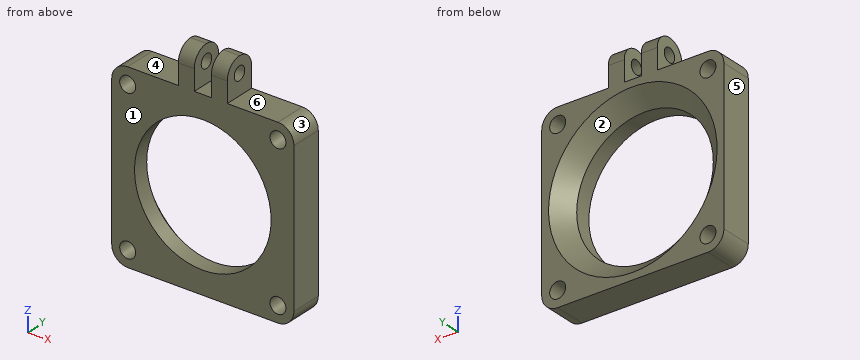
from build123d import *

# Parameters (mm, degrees)
BOSS_EXTRUDE1_DEPTH = 7
CUT_EXTRUDE2_REACH  = 31.138
SKETCH3_R           = 1.75
SKETCH7_W           = 3.5
SKETCH7_H           = 28
BOSS_EXTRUDE2_DEPTH = 7
CUT_EXTRUDE3_DEPTH  = 39.430334698
SKETCH9_R           = 1.5
CUT_EXTRUDE4_DEPTH  = 39.430334698
SKETCH13_R          = 15
CUT_EXTRUDE5_DEPTH  = 36.114099732


with BuildPart() as part:
    # Sketch1 → Boss-Extrude1 (new body)
    with BuildSketch(Plane(origin=(0, 0, 0), x_dir=(1, 0, 0), z_dir=(0, 1, 0))):
        with BuildLine():
            Line((-16.5, 20), (16.5, 20))
            ThreePointArc((16.5, 20), (18.974873734, 18.974873734), (20, 16.5))
            Line((20, 16.5), (20, -16.5))
            ThreePointArc((20, -16.5), (18.974873734, -18.974873734), (16.5, -20))
            Line((16.5, -20), (-16.5, -20))
            ThreePointArc((-16.5, -20), (-18.974873734, -18.974873734), (-20, -16.5))
            Line((-20, -16.5), (-20, 16.5))
            ThreePointArc((-20, 16.5), (-18.974873734, 18.974873734), (-16.5, 20))
        make_face()
    extrude(amount=BOSS_EXTRUDE1_DEPTH)

    # Sketch3 → Cut-Extrude2 (cut, up to next)
    with BuildSketch(Plane(origin=(0, 7, 0), x_dir=(1, 0, 0), z_dir=(0, 1, 0)), mode=Mode.PRIVATE) as cut_extrude2_sk1:
        with Locations(Location((-16.5, 16.5, 0), (0, 0, 270))):
            Circle(SKETCH3_R)
    cut_extrude2_tool1 = extrude(cut_extrude2_sk1.sketch, amount=-CUT_EXTRUDE2_REACH, mode=Mode.PRIVATE) & part.part
    # Sketch3 → Cut-Extrude2 (cut, up to next)
    with BuildSketch(Plane(origin=(0, 7, 0), x_dir=(1, 0, 0), z_dir=(0, 1, 0)), mode=Mode.PRIVATE) as cut_extrude2_sk2:
        with Locations(Location((16.5, 16.5, 0), (0, 0, 270))):
            Circle(SKETCH3_R)
    cut_extrude2_tool2 = extrude(cut_extrude2_sk2.sketch, amount=-CUT_EXTRUDE2_REACH, mode=Mode.PRIVATE) & part.part
    # Sketch3 → Cut-Extrude2 (cut, up to next)
    with BuildSketch(Plane(origin=(0, 7, 0), x_dir=(1, 0, 0), z_dir=(0, 1, 0)), mode=Mode.PRIVATE) as cut_extrude2_sk3:
        with Locations(Location((16.5, -16.5, 0), (0, 0, 270))):
            Circle(SKETCH3_R)
    cut_extrude2_tool3 = extrude(cut_extrude2_sk3.sketch, amount=-CUT_EXTRUDE2_REACH, mode=Mode.PRIVATE) & part.part
    # Sketch3 → Cut-Extrude2 (cut, up to next)
    with BuildSketch(Plane(origin=(0, 7, 0), x_dir=(1, 0, 0), z_dir=(0, 1, 0)), mode=Mode.PRIVATE) as cut_extrude2_sk4:
        with Locations(Location((-16.5, -16.5, 0), (0, 0, 270))):
            Circle(SKETCH3_R)
    cut_extrude2_tool4 = extrude(cut_extrude2_sk4.sketch, amount=-CUT_EXTRUDE2_REACH, mode=Mode.PRIVATE) & part.part
    add(cut_extrude2_tool1.solids().sort_by_distance((-16.5, 7, -16.5))[0], mode=Mode.SUBTRACT)
    add(cut_extrude2_tool2.solids().sort_by_distance((16.5, 7, -16.5))[0], mode=Mode.SUBTRACT)
    add(cut_extrude2_tool3.solids().sort_by_distance((16.5, 7, 16.5))[0], mode=Mode.SUBTRACT)
    add(cut_extrude2_tool4.solids().sort_by_distance((-16.5, 7, 16.5))[0], mode=Mode.SUBTRACT)

    # Sketch7 → Boss-Extrude2 (add)
    with BuildSketch(Plane.XZ):
        with Locations((3.625, 14)):
            Rectangle(SKETCH7_W, SKETCH7_H)
        with Locations((-3.625, 14)):
            Rectangle(SKETCH7_W, SKETCH7_H)
    extrude(amount=-BOSS_EXTRUDE2_DEPTH)

    # Sketch8 → Cut-Extrude3 (cut, through all)
    with BuildSketch(Plane(origin=(5.375, 0, 0), x_dir=(0, 0, -1), z_dir=(1, 0, 0))):
        with BuildLine():
            ThreePointArc((-28, 3.5), (-26.974873734, 5.974873734), (-24.5, 7))
            Line((-24.5, 7), (-28, 7))
            Line((-28, 7), (-28, 3.5))
        make_face()
        with BuildLine():
            ThreePointArc((-24.5, 0), (-26.974873734, 1.025126266), (-28, 3.5))
            Line((-28, 3.5), (-28, 0))
            Line((-28, 0), (-24.5, 0))
        make_face()
    extrude(amount=-CUT_EXTRUDE3_DEPTH, mode=Mode.SUBTRACT)

    # Sketch9 → Cut-Extrude4 (cut, through all)
    with BuildSketch(Plane(origin=(5.375, 0, 0), x_dir=(0, 0, -1), z_dir=(1, 0, 0))):
        with Locations((-24.5, 3.5)):
            Circle(SKETCH9_R)
    extrude(amount=-CUT_EXTRUDE4_DEPTH, mode=Mode.SUBTRACT)

    # Sketch13 → Cut-Extrude5 (cut, through all)
    with BuildSketch(Plane.XZ):
        with Locations(Location((0, 0, 0), (0, 0, 270))):
            Circle(SKETCH13_R)
    extrude(amount=-CUT_EXTRUDE5_DEPTH, mode=Mode.SUBTRACT)

    # Sketch14 → Cut-Revolve1 (revolve, cut)
    with BuildSketch(Plane(origin=(0, 0, 0), x_dir=(0, 0, -1), z_dir=(1, 0, 0))):
        Polygon((0, 0), (0, 7), (18.5, 7), (15, 3.5), (15, 0), align=None)
    revolve(axis=Axis((0, 7, 0), (0, -1, 0)), mode=Mode.SUBTRACT)


solid = part.part
For this review, take the finished solid that the model builds, in its own axes (mm). Face numbers are marked on the shaded views. A direction names the side the tool comes from. Round coordinates to 2 decimals unless told otherwise and drop trailing zeros. Write each loop counter-clockwise with the first axis right and the second up, starting at its lowest first coordinate (ties: lowest second). Pieces come first, ordered by that corner, then holes. Notation, with made-up numbers: M 51.5,-6 L 84.5,-6 A26 cw 84.5,26 Z; hole C 77.5,73 d9. An arc over 180 degrees is marked long. Write item = value, one per line. Start each with the question number.
(1) The part is to be moulded in two halves that separate along Z. For the marked faces 1, 2 and 3, say which applies: +Z half, -Z half, draft (parallel to the pull), parting line (faces both ways), or undercut.
(2) For line 1 along X through (y, z) = (3, -16.5); line 2 along X through (y, z) = (0.75, 0.5); line 3 along X through (y, z) = (4.5, 22) (3 decimals), list the stretches that pass through material, from the lowest coordinate up.
(3) For the marked faces 4, 5 and 6, list the 3-axis set-ups (+Z, -Z, +X, -X, +Y, -Y) from which the entire face can be reached by the end or side of a thin tool; tool diameter is ignored.
(4) We need section A-A (y = 2.75). Give the number of separate pieces and of enclosed holes in the cut face, then the cut area to 3 significant figures.
(5) We need section B-B (x = 0). Give the boundary of the cut face in (y, z), then the cut area to 4 significant figures.
(6) Clearance check with flat-ended pins moving along their axes: pin 1 Ø1.5 at (x, z) = (12.5, -12.5) entering from +Y; pin 2 Ø3 at (x, z) = (-5.5, -14.5) entering from -Y; pin 3 Ø3 at (x, z) = (-16.5, 16.5) entering from +Y; pin 4 Ø3.5 at (y, z) = (2, 25) entering from +X (3 decimals). State where each tip first meets the part, or that it passes through.
Results found:
q1.face_1 = draft
q1.face_2 = undercut
q1.face_3 = +Z half
q2.line_1 = -20 to -18.25, -14.75 to 14.75, 18.25 to 20
q2.line_2 = -20 to -14.99, 14.99 to 20
q2.line_3 = -5.375 to -1.875, 1.875 to 5.375
q3.face_4 = +Z, -X, +Y, -Y
q3.face_5 = +Z, -Z, -X, +Y, -Y
q3.face_6 = +Z, +X, +Y, -Y
q4.separate_pieces = 3
q4.enclosed_holes = 5
q4.area = 881 mm²
q5.outline = M 0,-20 L 7,-20 L 7,-18.5 L 3.5,-15 L 0,-15 Z; M 0,15 L 3.5,15 L 7,18.5 L 7,20 L 0,20 Z
q5.area = 57.75 mm²
q6.pin_1 = 6.93
q6.pin_2 = 0
q6.pin_3 = through
q6.pin_4 = 5.375
